Verification items for the finished model (mm, model axes). Face numbers are marked on the shaded views. A direction names the side the tool comes from. Give positions to 0.01 mm unless a question says otherwise; leave off trailing zeros. Order: outer loops, then holes, each group sorted by start corner. A loop starts at its lowest first (then second) coordinate and runs counter-clockwise, first axis right, second up. Notation, with made-up numbers: (10, 31.25) -> (64, 31.25) arc R24 cw to (64, 57.25) -> close; hole circle Ø2 at (79.5, 3.5). An arc over 180 degrees is marked (long way). Write each question's results on one line, items separated by ' | '. Start each with the question number.
1. Cross-section at A-A, the plane y = 0. Enter the section's corners in (x, z), then the cut area to 3 significant figures.
2. Cross-section at B-B, the plane z = 20.5. Enter the section's corners in (x, y), then the cut area to 3 significant figures.
3. Depth check by flat-ended pin: pin 1 Ø1.5 at (x, z) = (-6, 3) entering from +Y; pin 2 Ø1.5 at (x, y) = (-7.5, -0.5) entering from +Z; pin 3 Ø2 at (y, z) = (0, 14.5) entering from +X. Enter the tip coordinate at first touch or a pass-through.
4. Cross-section at C-C, the plane x = 8.75. Enter the section's corners in (y, z).
5. Material ranges on L1, parallel to X at y = 1.1, z = 2; L2, parallel to Z at x = 5, y = 0.5; L3, parallel to X at y = -0.15, z = 32, recorded low to high. Write a range as from..to.
6. Set-up check for the marked faces 1, 2, 3, 4 and 5: record each of +Z, -Z, +X, -X, +Y, -Y from which the full face is reachable in a straight line by a thin tool's end or side.
7. Cross-section at D-D, the plane y = -2. Enter the section's corners in (x, z).
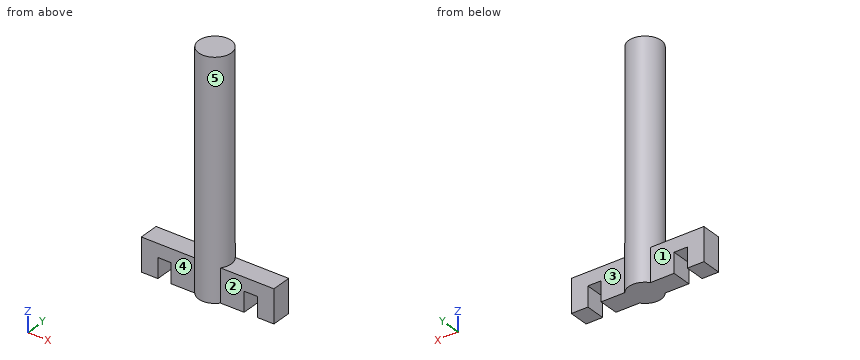
from build123d import *

# Parameters (mm, degrees)
SKETCH2_R           = 2.45
BOSS_EXTRUDE1_DEPTH = 35
SKETCH3_W           = 20
SKETCH3_H           = 3
BOSS_EXTRUDE2_DEPTH = 5
SKETCH4_W           = 2
SKETCH4_H           = 3
CUT_EXTRUDE1_DEPTH  = 3


with BuildPart() as part:
    # Sketch2 → Boss-Extrude1 (new body)
    with BuildSketch(Plane.XY):
        Circle(SKETCH2_R)
    extrude(amount=BOSS_EXTRUDE1_DEPTH)

    # Sketch3 → Boss-Extrude2 (add)
    with BuildSketch(Plane(origin=(0, 0, 0), x_dir=(-1, 0, 0), z_dir=(0, 0, -1))):
        Rectangle(SKETCH3_W, SKETCH3_H)
    extrude(amount=-BOSS_EXTRUDE2_DEPTH)

    # Sketch4 → Cut-Extrude1 (cut)
    with BuildSketch(Plane(origin=(0, 0, 0), x_dir=(-1, 0, 0), z_dir=(0, 0, -1))):
        with Locations((-6.5, 0)):
            Rectangle(SKETCH4_W, SKETCH4_H)
        with Locations((6.5, 0)):
            Rectangle(SKETCH4_W, SKETCH4_H)
    extrude(amount=-CUT_EXTRUDE1_DEPTH, mode=Mode.SUBTRACT)


solid = part.part
Results below:
1) outline: (-10, 0) -> (-7.5, 0) -> (-7.5, 3) -> (-5.5, 3) -> (-5.5, 0) -> (5.5, 0) -> (5.5, 3) -> (7.5, 3) -> (7.5, 0) -> (10, 0) -> (10, 5) -> (2.45, 5) -> (2.45, 35) -> (-2.45, 35) -> (-2.45, 5) -> (-10, 5) -> close | area: 235 mm²
2) outline: circle Ø4.9 at (0, 0) | area: 18.9 mm²
3) pin 1: stops at y = 1.5 | pin 2: stops at z = 5 | pin 3: stops at x = 2.45
4) outline: (-1.5, 0) -> (1.5, 0) -> (1.5, 5) -> (-1.5, 5) -> close
5) L1: x = -10..-7.5, -5.5..5.5, 7.5..10 | L2: z = 0..5 | L3: x = -2.45..2.45
6) face 1: +Z, -Z, -X, +Y | face 2: +Z, -Z, +X, -Y | face 3: +Z, -Z, +X, +Y | face 4: +Z, -Z, -X, -Y | face 5: +Z
7) outline: (-1.42, 0) -> (1.42, 0) -> (1.42, 35) -> (-1.42, 35) -> close
